from build123d import *

# Parameters (mm, degrees)
SKETCH1_W               = 45
SKETCH1_H               = 25
BOSS_EXTRUDE1_DEPTH     = 5
SKETCH2_W               = 5
SKETCH2_H               = 25
BOSS_EXTRUDE2_DEPTH     = 46
SKETCH3_W               = 45
SKETCH3_H               = 5
BOSS_EXTRUDE3_DEPTH     = 20
CHAMFER2_SIZE2          = 20
CHAMFER2_SIZE           = 28.562960135
CHAMFER3_SIZE2          = 20
CHAMFER3_SIZE           = 28.562960135
SKETCH4_W               = 5
SKETCH4_H               = 42
BOSS_EXTRUDE4_DEPTH     = 29
CUT_EXTRUDE1_DEPTH      = 76.213030786
CUT_EXTRUDE1_DEPTH_BACK = 76.213030786
SKETCH6_R               = 15
SKETCH7_W               = 46
SKETCH7_H               = 44
CUT_EXTRUDE2_DEPTH      = 76.213030786
SKETCH8_R               = 1.65
CUT_EXTRUDE3_DEPTH      = 76.213030786
SKETCH9_R               = 4
CUT_EXTRUDE4_DEPTH      = 76.213030786
FILLET1_R               = 5


with BuildPart() as part:
    # Sketch1 → Boss-Extrude1 (new body)
    with BuildSketch(Plane.XY):
        with Locations((22.5, 12.5)):
            Rectangle(SKETCH1_W, SKETCH1_H)
    extrude(amount=BOSS_EXTRUDE1_DEPTH)

    # Sketch2 → Boss-Extrude2 (add)
    with BuildSketch(Plane(origin=(0, 0, 0), x_dir=(-1, 0, 0), z_dir=(0, 0, -1))):
        with Locations((-22.5, 12.5)):
            Rectangle(SKETCH2_W, SKETCH2_H)
    extrude(amount=BOSS_EXTRUDE2_DEPTH)

    # Sketch3 → Boss-Extrude3 (add)
    with BuildSketch(Plane.XY.offset(5)):
        with Locations((22.5, 2.5)):
            Rectangle(SKETCH3_W, SKETCH3_H)
    extrude(amount=BOSS_EXTRUDE3_DEPTH)

    # Chamfer2
    chamfer2_edges = [part.edges().sort_by_distance(p)[0] for p in [
        (25, 12.5, 0),
    ]]
    chamfer2_side = [part.faces().sort_by_distance(p)[0] for p in [
        (25, 12.5, -0.4),
    ]]
    chamfer(chamfer2_edges, length=CHAMFER2_SIZE - 0.0001, length2=CHAMFER2_SIZE2 - 0.0001, reference=chamfer2_side[0])  # a hair under: the kernel refuses the full size

    # Chamfer3
    chamfer3_edges = [part.edges().sort_by_distance(p)[0] for p in [
        (20, 12.5, 0),
    ]]
    chamfer3_side = [part.faces().sort_by_distance(p)[0] for p in [
        (20, 12.5, -0.4),
    ]]
    chamfer(chamfer3_edges, length=CHAMFER3_SIZE - 0.0001, length2=CHAMFER3_SIZE2 - 0.0001, reference=chamfer3_side[0])  # a hair under: the kernel refuses the full size

    # Sketch4 → Boss-Extrude4 (add)
    with BuildSketch(Plane(origin=(0, 25, 0), x_dir=(1, 0, 0), z_dir=(0, 1, 0))):
        with Locations((22.5, 25)):
            Rectangle(SKETCH4_W, SKETCH4_H)
    extrude(amount=BOSS_EXTRUDE4_DEPTH)

    # Sketch6 → Cut-Extrude1 (cut, two sides: drawn at the far end of the back side and taken through both)
    with BuildSketch(Plane(origin=(25, 0, 0), x_dir=(0, 0, -1), z_dir=(1, 0, 0)).offset(-CUT_EXTRUDE1_DEPTH_BACK)):
        with Locations(Location((25, 33, 0), (0, 0, 283.740844537))):
            Circle(SKETCH6_R)
    extrude(amount=CUT_EXTRUDE1_DEPTH + CUT_EXTRUDE1_DEPTH_BACK, mode=Mode.SUBTRACT)

    # Sketch7 → Cut-Extrude2 (cut, through all)
    with BuildSketch(Plane.ZY.offset(-20)):
        with Locations((-23, 32)):
            Rectangle(SKETCH7_W, SKETCH7_H)
    extrude(amount=CUT_EXTRUDE2_DEPTH, mode=Mode.SUBTRACT)

    # Sketch8 → Cut-Extrude3 (cut, through all)
    with BuildSketch(Plane.ZY.offset(-20)):
        with Locations(Location((-40.5, 48.5, 0), (0, 0, 270))):
            Circle(SKETCH8_R)
        with Locations(Location((-9.5, 48.5, 0), (0, 0, 270))):
            Circle(SKETCH8_R)
        with Locations(Location((-9.5, 17.5, 0), (0, 0, 270))):
            Circle(SKETCH8_R)
        with Locations(Location((-40.5, 17.5, 0), (0, 0, 270))):
            Circle(SKETCH8_R)
    extrude(amount=-CUT_EXTRUDE3_DEPTH, mode=Mode.SUBTRACT)

    # Sketch9 → Cut-Extrude4 (cut, through all)
    with BuildSketch(Plane(origin=(25, 0, 0), x_dir=(0, 0, -1), z_dir=(1, 0, 0))):
        with Locations((9.5, 17.5)):
            Circle(SKETCH9_R)
    extrude(amount=CUT_EXTRUDE4_DEPTH, mode=Mode.SUBTRACT)

    # Fillet1
    fillet1_edges = [part.edges().sort_by_distance(p)[0] for p in [
        (22.5, 0, -46),
        (22.5, 54, -4),
        (22.5, 54, -46),
    ]]
    fillet(fillet1_edges, radius=FILLET1_R)


solid = part.part
Input: part model. Units: mm. Frame: model coordinates. A direction names the side the tool comes from. Give positions to 0.01 mm unless a question says otherwise; leave off trailing zeros. Order: outer loops, then holes, each group sorted by start corner. A loop starts at its lowest first (then second) coordinate and runs counter-clockwise, first axis right, second up. Notation, with made-up numbers: (-4, 41) - (17, 41) arc R22 ccw to (17, 49) - close; hole circle Ø6 at (53.5, -13). An arc over 180 degrees is marked (long way). Write each question's results on one line, items separated by ' | '.
Item 1: Draft query along Z for faces 4 (the cylindrical face through (22.46, 50.15, -9.43)), 5 (the flat face through (35.14, 9.55, -14.08)), 6 (the flat face through (25, 27, -39)), 7 (the flat face through (22, 15, 5)). Return one class per face: released by +Z, released by -Z, zero draft, split by the parting line, or undercut.
A:
face 4: undercut | face 5: released by -Z | face 6: zero draft | face 7: released by +Z
Item 2: Material intervals for line 1 along Z through (x, y) = (22.6, 48.5); line 2 along Y through (x, z) = (29, -9.5); line 3 along Z through (x, y) = (23, 17), sorted ascending.
A:
line 1: z = -46 to -42.15, -38.85 to -11.15, -7.85 to -4 | line 2: y = 0 to 13.5, 21.5 to 25 | line 3: z = -46 to -42.07, -38.93 to -11.07, -7.93 to 5
Item 3: Section C-C (x = 33.5). Return loops of the section in (y, z).
A:
outline: (0, -16.42) - (20.69, -16.42) arc R15 cw to (25, -12.31) - (25, 5) - (5, 5) - (5, 25) - (0, 25) - close; hole circle Ø8 at (17.5, -9.5)
Item 4: Section B-B (z = -19). Return loops of the section in (x, y), and give its area (3 significant figures).
A:
outline: (13.3, 0) - (31.7, 0) - (31.7, 19.25) - (20, 19.25) - (20, 10) - (13.3, 10) - close; (20, 46.75) - (25, 46.75) - (25, 54) - (20, 54) - close | area: 328 mm^2
Item 5: Section D-D (x = 17.5). Return loops of the section in (y, z).
A:
outline: (0, -24.99) - (10, -24.99) - (10, 0) - (25, 0) - (25, 5) - (5, 5) - (5, 25) - (0, 25) - close
Item 6: Section A-A (y = 33). Return loops of the section in (x, z), and give its area (3 significant figures).
A:
outline: (20, -46) - (25, -46) - (25, -40) - (20, -40) - close; (20, -10) - (25, -10) - (25, -4) - (20, -4) - close | area: 60.0 mm^2
Item 7: Contact query for flat-ended pins moving along their axis: pin 1 Ø1 at (x, z) = (31.5, -17) entering from +Y; pin 2 Ø12 at (x, y) = (7.5, 30) entering from -Z; pin 3 Ø4 at (y, z) = (17.5, -40.5) entering from +X; pin 4 Ø3 at (y, z) = (48.5, -9.5) entering from +X. Output: stop coordinate, or through.
A:
pin 1: stops at y = 20.64 | pin 2: stops at z = 0 | pin 3: stops at x = 25 | pin 4: passes through
Item 8: Access query for faces 1 (the flat face through (10, 18, 0)), 2 (the flat face through (25, 15.8, -10.3)), 3 (the flat face through (45, 7, 4)). Directions: +Z, -Z, +X, -X, +Y, -Y. A direction counts if a zero-diameter tool reaches every point of the face in a straight line with its end or side. Return the directions, or none.
A:
face 1: -Z, -X, +Y | face 2: +X | face 3: +Z, -Z, +X, +Y, -Y
